The listing builds one solid part. Answer for the finished solid, in the listing's coordinates (mm). Face numbers are marked on the shaded views. Coordinates: 2 decimals unless noted, no trailing zeros. Order: outer loops, then holes, each group sorted by start corner. A loop starts at its lowest first (then second) coordinate and runs counter-clockwise, first axis right, second up. Notation, with made-up numbers: M -34,27 L 25,27 A36 ccw 25,66 Z; hole C 20,29.5 d11. An arc over 180 degrees is marked long. One line per item, written item: value. Start each with the question number.
Q1. The part is cut by section B-B on z = 4.5. Give the vertices of the cut face in (x, y), then the cut area to 3 significant figures.
Q2. The part is cut by section A-A on y = 0. Give the vertices of the cut face in (x, z), then the cut area to 3 significant figures.
Q3. Each of these flat-tipped pins is pushed along its axis until it touches: pin 1 Ø16 at (x, y) = (2.5, 7.5) entering from +Z; pin 2 Ø5 at (x, z) = (-3, 5.5) entering from -Y; pin 3 Ø6 at (y, z) = (-8, 9) entering from -X; pin 4 Ø2 at (x, z) = (-7.5, 11.5) entering from -Y. Where does it stop, or does it pass through?
Q4. Straight lines are drawn through the part: line 1 along Y through (x, z) = (0, 11); line 2 along Y through (x, z) = (0, 7); line 3 along Z through (x, y) = (7, 6). For each, find the intervals that lie inside material, in ascending order. Write a range as [from, to].
Q5. Determine the mould class of the marked faces 1, 2 and 3 for opening direction X: pulls with the +X half, pulls with the -X half, needs draft (parallel to the pull), parting line crosses it, or undercut.
Q6. The part is cut by section D-D on z = 7. Give the vertices of the cut face in (x, y), then the cut area to 3 significant figures.
```python
from build123d import *

# Parameters (mm, degrees)
CHAMFER001_ANGLE = 3
CHAMFER001_SIZE  = 7
SKETCH001_W      = 10
SKETCH001_H      = 25.260876


with BuildPart() as part:
    # Sketch052 → Revolution001 (revolve)
    with BuildSketch(Plane.XZ):
        Polygon((0, 0), (16.25, 0), (16.25, 5), (15, 5), (15, 13), (0, 13), align=None)
    revolve(axis=Axis((0, 0, 0), (0, 0, 1)))

    # Chamfer001
    chamfer001_edges = [part.edges().sort_by_distance(p)[0] for p in [
        (-15, 0, 13),
    ]]
    chamfer001_side = part.faces().sort_by_distance((-15, 0, 9))[0]
    chamfer(chamfer001_edges, length=CHAMFER001_SIZE, angle=CHAMFER001_ANGLE, reference=chamfer001_side)

    # Sketch001 → Groove001 (revolve, cut)
    with BuildSketch(Plane.XZ):
        with Locations((5, 15.630438)):
            Rectangle(SKETCH001_W, SKETCH001_H)
    revolve(axis=Axis((0, 0, 0), (0, 0, 1)), mode=Mode.SUBTRACT)


solid = part.part
```
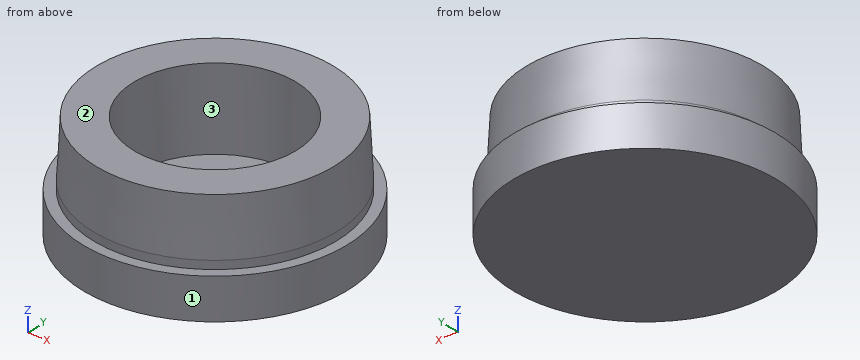
Output:
1. outline: C 0,0 d32.5; hole C 0,0 d20
1. area: 515 mm^2
2. outline: M -16.25,0 L 16.25,0 L 16.25,5 L 15,5 L 15,6 L 14.63,13 L 10,13 L 10,3 L -10,3 L -10,13 L -14.63,13 L -15,6 L -15,5 L -16.25,5 Z
2. area: 200 mm^2
3. pin 1: stops at z = 13
3. pin 2: stops at y = -16.24
3. pin 3: stops at x = -13.99
3. pin 4: stops at y = -13.2
4. line 1: y = [-14.74, -10], [10, 14.74]
4. line 2: y = [-14.95, -10], [10, 14.95]
4. line 3: z = [0, 3]
5. face 1: parting line crosses it
5. face 2: needs draft
5. face 3: undercut
6. outline: C 0,0 d29.9; hole C 0,0 d20
6. area: 388 mm^2
